```python
from build123d import *

# Parameters (mm, degrees)
SKETCH1_W           = 30
SKETCH1_H           = 60
BOSS_EXTRUDE1_DEPTH = 50
BOSS_EXTRUDE2_DEPTH = 45
SKETCH3_W           = 74.963778589
SKETCH3_H           = 76
SKETCH3_R           = 2
BOSS_EXTRUDE3_DEPTH = 4
SKETCH4_R           = 1.5
CUT_EXTRUDE1_DEPTH  = 5


with BuildPart() as part:
    # Sketch1 → Boss-Extrude1 (new body)
    with BuildSketch(Plane(origin=(0, 0, 0), x_dir=(1, 0, 0), z_dir=(0, 1, 0))):
        Rectangle(SKETCH1_W, SKETCH1_H)
    extrude(amount=BOSS_EXTRUDE1_DEPTH)

    # Sketch2 → Boss-Extrude2 (add)
    with BuildSketch(Plane(origin=(15, 0, 0), x_dir=(0, 0, -1), z_dir=(1, 0, 0))):
        with BuildLine():
            Line((-25.98102227, 30.006782085), (-30, 30.006782085))
            Line((-30, 30.006782085), (-30, 0))
            Line((-30, 0), (30, 0))
            Line((30, 0), (30, 30.006782085))
            Line((30, 30.006782085), (25.98102227, 30.006782085))
            ThreePointArc((25.98102227, 30.006782085), (0, 5), (-25.98102227, 30.006782085))
        make_face()
    extrude(amount=BOSS_EXTRUDE2_DEPTH)

    # Sketch3 → Boss-Extrude3 (add)
    with BuildSketch(Plane.XZ):
        with Locations((22.604342162, 0)):
            Rectangle(SKETCH3_W, SKETCH3_H)
        with Locations(Location((-11, 34, 0), (0, 0, 270))):
            Circle(SKETCH3_R, mode=Mode.SUBTRACT)
        with Locations(Location((56, 34, 0), (0, 0, 270))):
            Circle(SKETCH3_R, mode=Mode.SUBTRACT)
        with Locations(Location((56, -34, 0), (0, 0, 270))):
            Circle(SKETCH3_R, mode=Mode.SUBTRACT)
        with Locations(Location((-11, -34, 0), (0, 0, 270))):
            Circle(SKETCH3_R, mode=Mode.SUBTRACT)
    extrude(amount=-BOSS_EXTRUDE3_DEPTH)

    # Sketch4 → Cut-Extrude1 (cut)
    with BuildSketch(Plane(origin=(15, 0, 0), x_dir=(0, 0, -1), z_dir=(1, 0, 0))):
        with Locations((0, 31)):
            Circle(SKETCH4_R)
    extrude(amount=-CUT_EXTRUDE1_DEPTH, mode=Mode.SUBTRACT)


solid = part.part
```
The listing builds one solid part. Answer for the finished solid, in the listing's coordinates (mm). A direction names the side the tool comes from. Coordinates: 2 decimals unless noted, no trailing zeros. Loops run counter-clockwise (first coordinate to the right, second up) from the corner with the lowest first, then second, coordinate; pieces in that order, holes last. Notation, with made-up numbers: (-30.75, 18.5) -> (-15.75, 18.5) arc R27 cw to (-15.75, 52.5) -> close; hole circle Ø1 at (-32, -4). An arc over 180 degrees is marked (long way). Return JSON: item names as keys, results as strings. Group by question number.
(1) A cutting plane is placed at D-D on x = 45.5. Write down the section's boundary in (y, z).
(2) A cutting plane is placed at A-A on z = -34. Write down the section's boundary in (x, y), and give its area (3 significant figures).
(3) Given pin 1 Ø15 at (x, y) = (17.5, 16.5) entering from +Z; pin 2 Ø4.5 at (y, z) = (1.5, 33) entering from -X; pin 3 Ø1 at (x, y) = (7, 39) entering from -Z, each flat-ended and moving along its own axis, determine where each tip first touches the part or whether it passes through.
(4) Determine the mould class of faces 1 (the flat face through (14, 25, -30)), 2 (the cylindrical face through (12.54, 32.01, 1.11)), 3 (the flat face through (37, 30.007, 28)) for opening direction Y: released by +Y, released by -Y, zero draft, split by the parting line, or undercut.
(5) A cutting plane is placed at C-C on y = 31. Write down the section's boundary in (x, z).
(6) A cutting plane is placed at B-B on x = 56. Write down the section's boundary in (y, z), and give its area (3 significant figures).
(7) Find the intervals of material crossed by probe 1 along X at (y, z) = (3, -34); probe 2 along Z at (x, y) = (13.5, 10); probe 3 along Y at (x, z) = (30.5, -1), in increasing order. Write a range as from..to.
(8) Which of the six approach directions +Z, -Z, +X, -X, +Y, -Y give full straight-line access (tool end or side, diameter ignored) to faces 4 (the flat face through (15, 27, 0)), 5 (the flat face through (22, 2, 38)), 6 (the flat face through (-14.878, 2, 34)), 7 (the flat face through (60, 5.6, 7.1)), 8 (the flat face through (-14.878, 2, -34))?
The answers:
{
 "1": {"outline": "(0, -38) -> (4, -38) -> (4, -30) -> (30.01, -30) -> (30.01, -25.98) arc R26 cw to (30.01, 25.98) -> (30.01, 30) -> (4, 30) -> (4, 38) -> (0, 38) -> close"},
 "2": {"outline": "(-14.88, 0) -> (-13, 0) -> (-13, 4) -> (-14.88, 4) -> close; (-9, 0) -> (54, 0) -> (54, 4) -> (-9, 4) -> close; (58, 0) -> (60.09, 0) -> (60.09, 4) -> (58, 4) -> close", "area": "268 mm^2"},
 "3": {"pin 1": "stops at z = 30", "pin 2": "stops at x = -14.88", "pin 3": "stops at z = -30"},
 "4": {"face 1": "zero draft", "face 2": "undercut", "face 3": "released by +Y"},
 "5": {"outline": "(-15, -30) -> (15, -30) -> (15, -1.5) -> (10, -1.5) -> (10, 1.5) -> (15, 1.5) -> (15, 30) -> (-15, 30) -> close"},
 "6": {"outline": "(0, -38) -> (4, -38) -> (4, -36) -> (0, -36) -> close; (0, -32) -> (4, -32) -> (4, -30) -> (30.01, -30) -> (30.01, -25.98) arc R26 cw to (30.01, 25.98) -> (30.01, 30) -> (4, 30) -> (4, 32) -> (0, 32) -> close; (0, 36) -> (4, 36) -> (4, 38) -> (0, 38) -> close", "area": "822 mm^2"},
 "7": {"probe 1": "x = -14.88..-13, -9..54, 58..60.09", "probe 2": "z = -30..30", "probe 3": "y = 0..5.02"},
 "8": {"face 4": "+X, +Y", "face 5": "+Z, +X, -X, +Y, -Y", "face 6": "+Z, -X, +Y, -Y", "face 7": "+Z, -Z, +X, +Y", "face 8": "-Z, -X, +Y, -Y"}
}
